Build history of the part. All positions in model axes, mm. A direction names the side the tool comes from. Give positions to 0.01 mm unless a question says otherwise; leave off trailing zeros. Write each loop counter-clockwise with the first axis right and the second up, starting at its lowest first coordinate (ties: lowest second). Pieces come first, ordered by that corner, then holes. Notation, with made-up numbers: (-19.5, 1.25) -> (28.5, 1.25) arc R25 ccw to (28.5, 26.25) -> close; hole circle Ø7 at (54, 50). An arc over 180 degrees is marked (long way). Put each result on its own line as item: value.
Solid Edge part; units mm, degrees
sketch "Sketch1" plane through (0, 0, 0) normal (0, -1, 0) x (1, 0, 0)
  line L0 (-42.5, -7.5) -> (42.5, -7.5)
  line L1 (42.5, 7.5) -> (-42.5, 7.5)
  arc A0 (42.5, 7.5) -> (42.5, -7.5) centre (42.5, 0) cw
  arc A1 (-42.5, -7.5) -> (-42.5, 7.5) centre (-42.5, 0) cw
extrude "Protrusion1" add sketch "Sketch1" against normal blind 5
sketch "Sketch2" plane through (0, 0, 0) normal (0, -1, 0) x (1, 0, 0)
  circle A0 centre (-42.5, 0) radius 7.5
  circle A1 centre (42.5, 0) radius 7.5
extrude "ExtrudedProtrusion_3" add sketch "Sketch2" against normal blind 25
sketch "Sketch3" plane through (0, 0, 0) normal (0, -1, 0) x (1, 0, 0)
  circle A0 centre (0, 0) radius 7.5
extrude "ExtrudedProtrusion_5" add sketch "Sketch3" along normal blind 4
properties material "Stainless steel"
1) Slice it at B-B (x = -40). Write the cut outline in (y, z).
Filled sheet:
outline: (0, -7.5) -> (5, -7.5) -> (5, -7.07) -> (25, -7.07) -> (25, 7.07) -> (5, 7.07) -> (5, 7.5) -> (0, 7.5) -> close
2) Slice it at C-C (y = 1.5). Write the cut outline in (x, z).
Filled sheet:
outline: (-42.5, -7.5) -> (42.5, -7.5) arc R7.5 ccw to (42.5, 7.5) -> (-42.5, 7.5) arc R7.5 ccw to start
3) Pin check, flat tips, straight feed: pin 1 (4.5 mm diameter, centred on x = 26.5, z = 1, fed in from -Y); pin 2 (3 mm diameter, centred on x = 10, z = -4, fed in from +Y); pin 3 (5 mm diameter, centred on y = 14, z = 3, fed in from +X). Stop position of each tip, or through.
Filled sheet:
pin 1: y = 0
pin 2: y = 5
pin 3: x = 49.98
4) Tool access for faces 1 (the cylindrical face through (-50, 12, 0)), 2 (the flat face through (1, 2, 7.5)), 3 (the cylindrical face through (-7.493, -1.972, -0.33)): list every direction of +Z, -Z, +X, -X, +Y, -Y with a clear straight run to the whole face (end or side of a thin tool).
Filled sheet:
face 1: +Y
face 2: +Z, +X, -X, +Y, -Y
face 3: -Y
5) Slice it at A-A (y = 17.75). Write the cut outline in (x, z).
Filled sheet:
outline: circle Ø15 at (-42.5, 0); circle Ø15 at (42.5, 0)
6) Slice it at D-D (x = -10.5). Write the cut outline in (y, z).
Filled sheet:
outline: (0, -7.5) -> (5, -7.5) -> (5, 7.5) -> (0, 7.5) -> close
7) Wall check: L1, parallel to X at y = 17.5, z = 0.25; L2, parallel to Y at x = 6, z = -2; L3, parallel to Y at x = 22, z = -1.75. Give the ranges that are in metal, low to high.
Filled sheet:
L1: -50 to -35, 35 to 50
L2: -4 to 5
L3: 0 to 5
